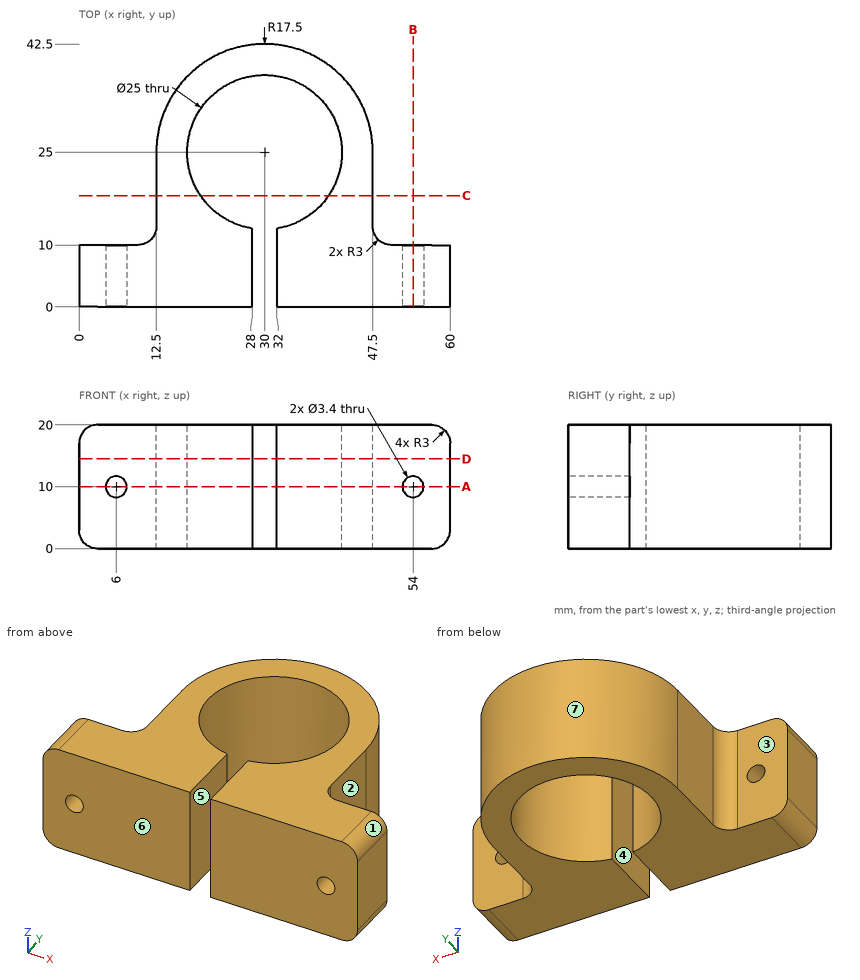
Study the drawing (mm; zero at the part's minimum x, y, z) and answer. A direction names the side the tool comes from. Give positions to 0.01 mm unless a question says otherwise; leave off trailing zeros. Write each loop counter-clockwise with the first axis right and the second up, starting at its lowest first coordinate (ties: lowest second). Pieces come first, ordered by that corner, then holes.
Item 1: Section B-B, the plane x = 54 is taken. Write down the section's boundary in (y, z).
Item 2: Section D-D, the plane z = 14.5 is taken. Write down the section's boundary in (x, y), plus the area to 3 significant figures.
Item 3: Find the intervals of material crossed by line 1 along X through (y, z) = (25, 9.75); line 2 along X through (y, z) = (7.5, 16); line 3 along Z through (x, y) = (54, 4.25), in increasing order.
Item 4: Which of the six approach directions +Z, -Z, +X, -X, +Y, -Y give full straight-line access (tool end or side, diameter ignored) to the marked faces 1, 2 and 3?
Item 5: Flat-ended cylindrical pins translate along their axes: P1, Ø3, axis at x = 53, z = 6.5, coming from the +Y side; P2, Ø1, axis at y = 25, z = 8.5, coming from the +X side; P3, Ø6, axis at x = 19.5, z = 13, coming from the +Y side; P4, Ø4, axis at y = 9.5, z = 12, coming from the -X side. Find the tip coordinate at first contact, or state that the pin passes through.
Item 6: Determine the mould class of the marked faces 4, 5, 6 and 7 for opening direction X: released by +X, released by -X, zero draft, split by the parting line, or undercut.
Item 7: Section C-C, the plane y = 18 is taken. Write down the section's boundary in (x, z).
Item 8: Section A-A, the plane z = 10 is taken. Write down the section's boundary in (x, y).
Completed:
1. outline: (0, 0) - (10, 0) - (10, 8.3) - (0, 8.3) - close; (0, 11.7) - (10, 11.7) - (10, 20) - (0, 20) - close
2. outline: (0, 0) - (28, 0) - (28, 12.66) arc R12.5 cw (long way) to (32, 12.66) - (32, 0) - (60, 0) - (60, 10) - (50.5, 10) arc R3 cw to (47.5, 13) - (47.5, 25) arc R17.5 ccw to (12.5, 25) - (12.5, 13) arc R3 cw to (9.5, 10) - (0, 10) - close
2. area: 1,070 mm2
3. line 1: x = 12.5 to 17.5, 42.5 to 47.5
3. line 2: x = 0 to 28, 32 to 60
3. line 3: z = 0 to 8.3, 11.7 to 20
4. face 1: +Z, +X, +Y, -Y
4. face 2: +Z, -Z, +X, +Y
4. face 3: +Z, -Z, -X, +Y
5. P1: stops at y = 10
5. P2: stops at x = 47.5
5. P3: stops at y = 40.81
5. P4: stops at x = 0
6. face 4: undercut
6. face 5: undercut
6. face 6: zero draft
6. face 7: split by the parting line
7. outline: (12.5, 0) - (19.64, 0) - (19.64, 20) - (12.5, 20) - close; (40.36, 0) - (47.5, 0) - (47.5, 20) - (40.36, 20) - close
8. outline: (0, 0) - (4.3, 0) - (4.3, 10) - (0, 10) - close; (7.7, 0) - (28, 0) - (28, 12.66) arc R12.5 cw (long way) to (32, 12.66) - (32, 0) - (52.3, 0) - (52.3, 10) - (50.5, 10) arc R3 cw to (47.5, 13) - (47.5, 25) arc R17.5 ccw to (12.5, 25) - (12.5, 13) arc R3 cw to (9.5, 10) - (7.7, 10) - close; (55.7, 0) - (60, 0) - (60, 10) - (55.7, 10) - close
